Input: part model. Units: mm. Frame: model coordinates. Face numbers are marked on the shaded views. A direction names the side the tool comes from. Coordinates: 2 decimals unless noted, no trailing zeros. Write each loop counter-clockwise with the first axis right and the second up, starting at its lowest first coordinate (ties: lowest second). Pieces come first, ordered by that corner, then holes. Notation, with made-up numbers: (0, -8) -> (53, -8) arc R14 ccw to (53, 10) -> close; hole circle Ø9 at (-40, 3). An arc over 180 degrees is marked (long way). Use one line per item in the form item = value. Start each with the question number.
(1) Ray query, line 1 along Z through (x, y) = (1.75, -3); line 2 along Y through (x, z) = (2.25, -20); line 3 along Z through (x, y) = (5.25, 1.75). Return the intervals inside material, ascending.
(2) Set-up query: the marked faces 4, 5 and 6. Return all of +Z, -Z, +X, -X, +Y, -Y with unobstructed straight access to the full face (end or side cutting, diameter ignored); none if empty.
(3) Pull-direction query (Z, two-part tool) for the marked faces 1, 2 and 3; classes: released by +Z, released by -Z, zero draft, split by the parting line, or undercut.
(4) Cut plane A-A on z = -67. Return the cut outline in (x, y) (3 decimals), plus the area to 3 significant figures.
(5) First-contact query: pin 1 (3 mm diameter, centred on x = 1, y = 0.5, fed in from -Z); pin 2 (4.5 mm diameter, centred on x = -1, z = -2.5, fed in from -Y); pin 3 (6.5 mm diameter, centred on x = 0, z = -5, fed in from +Y) (3 decimals); pin 4 (6.5 mm diameter, centred on x = -1, z = -30.5, fed in from +Y). Flat tips, straight axial feed; report the tip coordinate or a pass-through.
(6) Cut plane D-D on z = -51.5. Return the cut outline in (x, y), plus the area to 3 significant figures.
```python
from build123d import *

# Parameters (mm, degrees)
F1_DEPTH = 65.95
F3_DEPTH = 7.25
F5_DEPTH = 2
F8_DEPTH = 2
F9_SIZE  = 0.5
F10_SIZE = 2.12499


# Not quite as in the source:
# - a fillet or chamfer is up to 0.001 mm smaller than in the source, because OpenCascade refuses the exact size


with BuildPart() as f1:
    # F0 (on Top) → F1 (new body)
    with BuildSketch(Plane.XY):
        Polygon((-2.8867513459, -5), (2.8867513459, -5), (5.7735026919, 0), (2.8867513459, 5), (-2.8867513459, 5), (-5.7735026919, 0), align=None)
    extrude(amount=-F1_DEPTH)



with BuildPart() as f3:
    # F2 (on face) → F3 (new body)
    with BuildSketch(Plane(origin=(0, 0, -65.95), x_dir=(1, 0, 0), z_dir=(0, 0, -1))):
        Polygon((4.113620668, 7.125), (-4.113620668, 7.125), (-8.227241336, 0), (-4.113620668, -7.125), (4.113620668, -7.125), (8.227241336, 0), align=None)
        Polygon((2.9589201296, 5.125), (5.9178402592, 0), (2.9589201296, -5.125), (-2.9589201296, -5.125), (-5.9178402592, 0), (-2.9589201296, 5.125), align=None, mode=Mode.SUBTRACT)
    extrude(amount=F3_DEPTH)


with BuildPart() as f1_1:
    add(f1.part)

    add(f3.part)  # F5 merges F3
    # F4 (on face) → F5 (join)
    with BuildSketch(Plane.XY.offset(-65.95)):
        Polygon((-8.227241336, 0), (-4.113620668, -7.125), (4.113620668, -7.125), (8.227241336, 0), (4.113620668, 7.125), (-4.113620668, 7.125), align=None)
    extrude(amount=F5_DEPTH)

    # F7 (on offset) → F8 (join)
    with BuildSketch(Plane.XY.offset(-7)):
        Polygon((-8.227241336, 0), (-4.113620668, -7.125), (4.113620668, -7.125), (8.227241336, 0), (4.113620668, 7.125), (-4.113620668, 7.125), align=None)
    extrude(amount=-F8_DEPTH)

    # F9
    f9_edges = [f1_1.edges().sort_by_distance(p)[0] for p in [
        (-4.330127, -2.5, 0),
        (0, -5, 0),
        (4.330127, -2.5, 0),
        (4.330127, 2.5, 0),
        (0, 5, 0),
        (-4.330127, 2.5, 0),
        (-4.43838, 2.5625, -73.2),
        (-4.43838, -2.5625, -73.2),
        (0, -5.125, -73.2),
        (4.43838, -2.5625, -73.2),
        (4.43838, 2.5625, -73.2),
        (0, 5.125, -73.2),
    ]]
    chamfer(f9_edges, length=F9_SIZE)

    # F10 (size 2.125 in the source; OpenCascade refuses exactly that, so slightly less here)
    f10_edges = [f1_1.edges().sort_by_distance(p)[0] for p in [
        (0, 5, -63.95),
        (-4.330127, 2.5, -63.95),
        (-4.330127, -2.5, -63.95),
        (0, -5, -63.95),
        (4.330127, -2.5, -63.95),
        (4.330127, 2.5, -63.95),
        (-4.330127, 2.5, -9),
        (0, 5, -9),
        (-4.330127, -2.5, -9),
        (0, -5, -9),
        (4.330127, -2.5, -9),
        (4.330127, 2.5, -9),
    ]]
    chamfer(f10_edges, length=F10_SIZE)


solid = f1_1.part
```
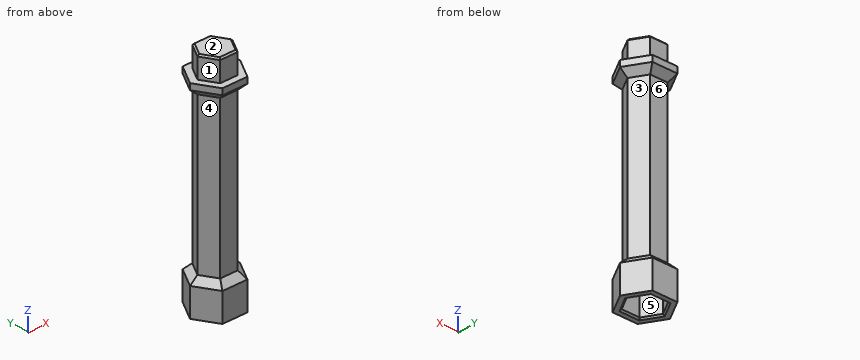
Values:
q1.line_1 = -65.95 to 0
q1.line_2 = -5 to 5
q1.line_3 = -73 to -62.25, -10.7 to -7
q2.face_4 = -X, -Y
q2.face_5 = -Z
q2.face_6 = +X, -X, +Y
q3.face_1 = zero draft
q3.face_2 = released by +Z
q3.face_3 = undercut
q4.outline = (-8.227, 0) -> (-4.114, -7.125) -> (4.114, -7.125) -> (8.227, 0) -> (4.114, 7.125) -> (-4.114, 7.125) -> close; hole (-5.918, 0) -> (-2.959, -5.125) -> (2.959, -5.125) -> (5.918, 0) -> (2.959, 5.125) -> (-2.959, 5.125) -> close
q4.area = 84.9 mm2
q5.pin_1 = -65.95
q5.pin_2 = -5
q5.pin_3 = 7.125
q5.pin_4 = 5
q6.outline = (-5.77, 0) -> (-2.89, -5) -> (2.89, -5) -> (5.77, 0) -> (2.89, 5) -> (-2.89, 5) -> close
q6.area = 86.6 mm2
